```python
from build123d import *

# Parameters (mm, degrees)
SKETCH1_R           = 5
SKETCH1_R_2         = 1.75
BOSS_EXTRUDE1_DEPTH = 6
CUT_EXTRUDE1_REACH  = 8
SKETCH2_R           = 1.25


with BuildPart() as part:
    # Sketch1 → Boss-Extrude1 (new body)
    with BuildSketch(Plane.XY):
        Polygon((348.916937196, 226.998518154), (348.916937196, 260.998518154), (301.716937196, 260.998518154), (301.716937196, 226.998518154), (316.850270529, 226.998518154), (316.850270529, 221.04907787), (333.783603862, 221.04907787), (333.783603862, 226.998518154), align=None)
        with Locations((325.316937196, 243.398518154)):
            Circle(SKETCH1_R, mode=Mode.SUBTRACT)
        with Locations((331.123946249, 248.901121707)):
            Circle(SKETCH1_R_2, mode=Mode.SUBTRACT)
        with Locations((319.814333643, 249.205527207)):
            Circle(SKETCH1_R_2, mode=Mode.SUBTRACT)
        with Locations((319.509928143, 237.895914601)):
            Circle(SKETCH1_R_2, mode=Mode.SUBTRACT)
        with Locations((330.819540748, 237.591509101)):
            Circle(SKETCH1_R_2, mode=Mode.SUBTRACT)
    extrude(amount=BOSS_EXTRUDE1_DEPTH)

    # Sketch2 → Cut-Extrude1 (cut, up to next)
    with BuildSketch(Plane.XY.offset(6), mode=Mode.PRIVATE) as cut_extrude1_sk1:
        with Locations((317.696937196, 256.998518154)):
            Circle(SKETCH2_R)
    cut_extrude1_tool1 = extrude(cut_extrude1_sk1.sketch, amount=-CUT_EXTRUDE1_REACH, mode=Mode.PRIVATE) & part.part
    add(cut_extrude1_tool1.solids().sort_by_distance((317.696937, 256.998518, 6))[0], mode=Mode.SUBTRACT)
    # Sketch2 → Cut-Extrude1 (cut, up to next)
    with BuildSketch(Plane.XY.offset(6), mode=Mode.PRIVATE) as cut_extrude1_sk2:
        with Locations((332.936937196, 256.998518154)):
            Circle(SKETCH2_R)
    cut_extrude1_tool2 = extrude(cut_extrude1_sk2.sketch, amount=-CUT_EXTRUDE1_REACH, mode=Mode.PRIVATE) & part.part
    add(cut_extrude1_tool2.solids().sort_by_distance((332.936937, 256.998518, 6))[0], mode=Mode.SUBTRACT)


solid = part.part
```
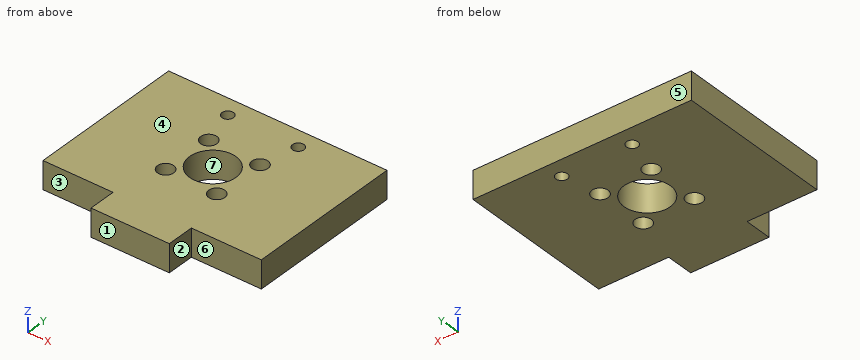
Input: part model. Units: mm. Frame: model coordinates. Face numbers are marked on the shaded views. A direction names the side the tool comes from. Give positions to 0.01 mm unless a question says otherwise; leave off trailing zeros. Order: outer loops, then holes, each group sorted by start corner. A loop starts at its lowest first (then second) coordinate and runs counter-clockwise, first axis right, second up. Notation, with made-up numbers: M -37.75,0.25 L -4.75,0.25 A8 ccw -4.75,11.25 Z; hole C 69.5,23 d5. An arc over 180 degrees is marked long. Return JSON: item names as keys, results as strings.
1) Section query C-C on z = 5.2. Output: boundary loops of the cut face in (x, y).
Taken from the geometry:
{"outline": "M 301.72,227 L 316.85,227 L 316.85,221.05 L 333.78,221.05 L 333.78,227 L 348.92,227 L 348.92,261 L 301.72,261 Z; hole C 317.7,257 d2.5; hole C 319.51,237.9 d3.5; hole C 319.81,249.21 d3.5; hole C 325.32,243.4 d10; hole C 330.82,237.59 d3.5; hole C 331.12,248.9 d3.5; hole C 332.94,257 d2.5"}
2) Contact query for flat-ended pins moving along their axis: pin 1 (3 mm diameter, centred on x = 332.94, y = 257, fed in from -Z); pin 2 (3 mm diameter, centred on y = 224.5, z = 2, fed in from +X); pin 3 (1.8 mm diameter, centred on x = 338, z = 4, fed in from -Y); pin 4 (8 mm diameter, centred on x = 325.32, y = 243.4, fed in from -Z) (3 decimals). Output: stop coordinate, or through.
Taken from the geometry:
{"pin 1": "stops at z = 0", "pin 2": "stops at x = 333.78", "pin 3": "stops at y = 227", "pin 4": "passes through"}
3) Section query A-A on x = 319.5. Output: boundary loops of the cut face in (y, z), and give its area (3 significant figures).
Taken from the geometry:
{"outline": "M 221.05,0 L 236.15,0 L 236.15,6 L 221.05,6 Z; M 239.65,0 L 247.48,0 L 247.48,6 L 239.65,6 Z; M 250.93,0 L 261,0 L 261,6 L 250.93,6 Z", "area": "198 mm2"}
4) Line query: L1, parallel to X at y = 250, z = 4.8; L2, parallel to Y at x = 320, z = 0.55; L3, parallel to Y at x = 321, z = 3.5. Output: solid intervals per line, ascending. Write a range as [from, to].
Taken from the geometry:
{"L1": "x = [301.72, 318.26], [321.37, 329.76], [332.49, 348.92]", "L2": "y = [221.05, 236.22], [239.58, 247.47], [250.95, 261]", "L3": "y = [221.05, 236.98], [238.81, 240.88], [245.92, 247.92], [250.49, 261]"}
5) Section query D-D on x = 312. Output: boundary loops of the cut face in (y, z), and give its area (3 significant figures).
Taken from the geometry:
{"outline": "M 227,0 L 261,0 L 261,6 L 227,6 Z", "area": "204 mm2"}
6) Access query for the marked faces 1, 2 and 3. Directions: +Z, -Z, +X, -X, +Y, -Y. A direction counts if a zero-diameter tool reaches every point of the face in a straight line with its end or side. Return the directions, or none.
Taken from the geometry:
{"face 1": "+Z, -Z, +X, -X, -Y", "face 2": "+Z, -Z, +X, -Y", "face 3": "+Z, -Z, -X, -Y"}
7) Mould query, pull axis Y, two halves, no side actions, for the marked faces 4, 5, 6 and 7. Classes: released by +Y, released by -Y, zero draft, split by the parting line, or undercut.
Taken from the geometry:
{"face 4": "zero draft", "face 5": "released by +Y", "face 6": "released by -Y", "face 7": "undercut"}
8) Section query B-B on y = 241. Output: boundary loops of the cut face in (x, z).
Taken from the geometry:
{"outline": "M 301.72,0 L 320.93,0 L 320.93,6 L 301.72,6 Z; M 329.7,0 L 348.92,0 L 348.92,6 L 329.7,6 Z"}
